Geometry: see drawing. Coordinates: mm, zero at the bounding-box minimum. A direction names the side the tool comes from. Coordinates: 2 decimals unless noted, no trailing zeros. Write each loop counter-clockwise with the first axis right and the second up, starting at its lowest first coordinate (ties: lowest second). Pieces come first, ordered by that corner, then holes. Notation, with made-up numbers: (-3.75, 9) - (16.25, 9) arc R32 cw to (16.25, 47) - close; hole circle Ø1 at (49, 43.5). An arc over 180 degrees is marked (long way). One line per question, with ' | ' between items. Start each with the question number.
1) Section query D-D on x = 113.5. Return loops of the section in (y, z), and give its area (3 significant figures).
2) Line query: line 1 (X direction, y = 12.5, z = 27); line 2 (X direction, y = 15.5, z = 32.5); line 3 (X direction, y = 9, z = 19.5). Output: solid intervals per line, ascending.
3) Section query B-B on x = 191. Return loops of the section in (y, z).
4) First-contact query: P1, Ø1, axis at x = 108, z = 42, coming from the -Y side; P2, Ø1.5, axis at x = 108.5, z = 38, coming from the +Y side; P3, Ø10, axis at y = 6, z = 14, coming from the +X side; P4, Ø10, axis at x = 196.5, y = 3, coming from the -Z side. Flat tips, straight axial feed; report the tip coordinate or a pass-through.
5) Reachability of the marked faces 1, 2 and 3 from +Z, -Z, +X, -X, +Y, -Y: full face, straight path, thin tool, end or side. Return the list, or none.
6) Section query C-C on z = 54.5. Return loops of the section in (x, y), and give its area (3 significant figures).
7) Draft query along X for the marked faces 4, 5 and 6. Return one class per face: released by +X, released by -X, zero draft, split by the parting line, or undercut.
8) Section query A-A on y = 17.75. Return loops of the section in (x, z).
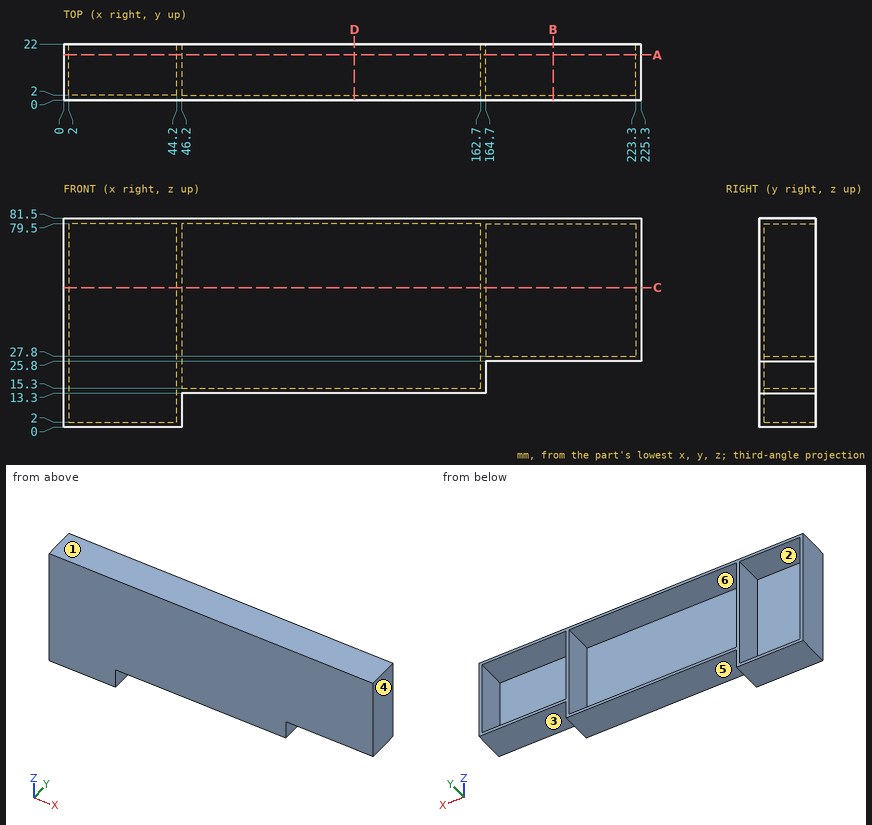
Answer key:
1) outline: (0, 13.3) - (22, 13.3) - (22, 15.3) - (2, 15.3) - (2, 79.5) - (22, 79.5) - (22, 81.5) - (0, 81.5) - close | area: 216 mm²
2) line 1: 0 to 2, 44.2 to 46.2, 162.7 to 225.3 | line 2: 0 to 2, 44.2 to 46.2, 162.7 to 164.7, 223.3 to 225.3 | line 3: 0 to 2, 44.2 to 46.2, 162.7 to 164.7
3) outline: (0, 25.8) - (22, 25.8) - (22, 27.8) - (2, 27.8) - (2, 79.5) - (22, 79.5) - (22, 81.5) - (0, 81.5) - close
4) P1: y = 0 | P2: y = 2 | P3: x = 164.7 | P4: z = 25.8
5) face 1: +Z, +X, -X, +Y, -Y | face 2: +Y | face 3: -Z, +X, +Y, -Y
6) outline: (0, 0) - (225.3, 0) - (225.3, 22) - (223.3, 22) - (223.3, 2) - (164.7, 2) - (164.7, 22) - (162.7, 22) - (162.7, 2) - (46.2, 2) - (46.2, 22) - (44.2, 22) - (44.2, 2) - (2, 2) - (2, 22) - (0, 22) - close | area: 611 mm²
7) face 4: released by +X | face 5: zero draft | face 6: undercut
8) outline: (0, 0) - (46.2, 0) - (46.2, 13.3) - (164.7, 13.3) - (164.7, 25.8) - (225.3, 25.8) - (225.3, 81.5) - (0, 81.5) - close; hole (2, 2) - (44.2, 2) - (44.2, 79.5) - (2, 79.5) - close; hole (46.2, 15.3) - (162.7, 15.3) - (162.7, 79.5) - (46.2, 79.5) - close; hole (164.7, 27.8) - (223.3, 27.8) - (223.3, 79.5) - (164.7, 79.5) - close
